Can you work these out from the model? Positions are in its coordinate system, mm. Face numbers are marked on the shaded views. A direction names the side the tool comes from. Give positions to 0.01 mm unless a question says otherwise; leave off trailing zeros. Loops run counter-clockwise (first coordinate to the right, second up) from the corner with the lowest first, then second, coordinate; pieces in that order, holes last. Notation, with made-up numbers: (83, 41.25) - (119, 41.25) arc R18 cw to (119, 50.25) - close; hole circle Ø11 at (61, 20). An arc over 180 degrees is marked (long way). Answer as a JSON object with one key per item and string values. Group by question number.
Item 1: Suppose I cut it at D-D on y = 4. Write out the boundary of the cut face in (x, z).
Item 2: Please list where these lines run through material, in increasing order: L1, parallel to Y at x = 0.5, z = 7.5; L2, parallel to Y at x = -5, z = 3.75; L3, parallel to X at y = 0, z = 8.75.
Item 3: Will these pins go through, and if not, where does the flat tip stop? pin 1 (8 mm diameter, centred on x = 14.5, y = 14, fed in from +Z); pin 2 (2 mm diameter, centred on x = -12, z = 2, fed in from +Y); pin 3 (5 mm diameter, centred on y = 20, z = 4.5, fed in from +X).
Item 4: Suppose I cut it at A-A on y = 28. Write out the boundary of the cut face in (x, z).
Item 5: Which directions (+Z, -Z, +X, -X, +Y, -Y) give clear straight access to the entire face, cutting with the end or side of a thin tool? Please do the marked faces 1, 2 and 3.
Item 6: Thinking about a two-plate mould opening in X: for the marked faces 4, 5 and 6, which applies, pulls with the +X half, pulls with the -X half, needs draft (parallel to the pull), parting line crosses it, or undercut?
Item 7: Suppose I cut it at B-B on x = 17.5. Write out the boundary of the cut face in (y, z), and give its area (3 significant figures).
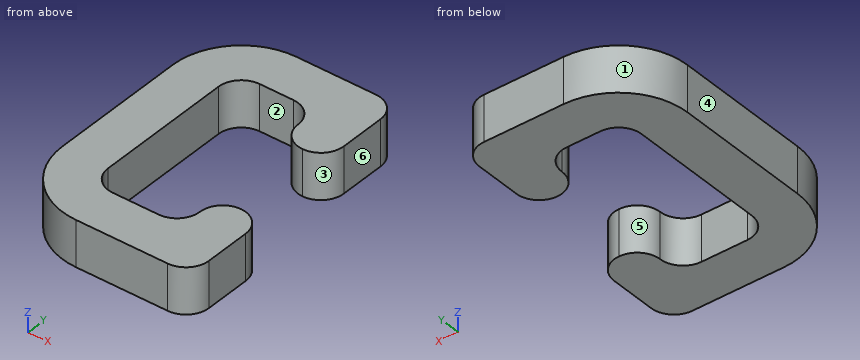
from build123d import *

# Parameters (mm, degrees)
F0_W     = 10
F0_H     = 10
F1_DEPTH = 10
F2_R     = 4.99999
F3_R     = 5
F4_R     = 5
F5_R     = 15


# Not quite as in the source:
# - a fillet or chamfer is up to 0.001 mm smaller than in the source, because OpenCascade refuses the exact size


with BuildPart() as f1:
    # F0 (on Top) → F1 (new body)
    with BuildSketch(Plane.XY):
        Polygon((10.8962109051, 41.5868479488), (10.8962109051, 31.5868479488), (10.8962109051, 21.5868479488), (20.8962109051, 21.5868479488), (20.8962109051, 41.5868479488), align=None)
        Polygon((-16.4567323537, 41.5868479488), (-16.4567323537, 31.5868479488), (-6.4567323537, 31.5868479488), (10.8962109051, 31.5868479488), (10.8962109051, 41.5868479488), align=None)
        Polygon((-6.4567323537, 31.5868479488), (-16.4567323537, 31.5868479488), (-16.4567323537, -18.4131520512), (-6.4567323537, -18.4131520512), (-6.4567323537, -8.4131520512), align=None)
        Polygon((13.5432676463, -8.4131520512), (-6.4567323537, -8.4131520512), (-6.4567323537, -18.4131520512), (23.5432676463, -18.4131520512), (23.5432676463, -8.4131520512), align=None)
        with Locations((18.5432676463, -3.4131520512)):
            Rectangle(F0_W, F0_H)
    extrude(amount=F1_DEPTH)

    # F2 (radius 5 in the source; OpenCascade refuses exactly that, so slightly less here)
    f2_edges = [f1.edges().sort_by_distance(p)[0] for p in [
        (13.543268, 1.586848, 5),
        (10.896211, 21.586848, 5),
        (10.896211, 31.586848, 5),
        (-6.456732, 31.586848, 5),
        (-6.456732, -8.413152, 5),
        (13.543268, -8.413152, 5),
    ]]
    fillet(f2_edges, radius=F2_R)

    # F3
    f3_edges = [f1.edges().sort_by_distance(p)[0] for p in [
        (23.543268, 1.586848, 5),
        (20.896211, 21.586848, 5),
    ]]
    fillet(f3_edges, radius=F3_R)

    # F4
    f4_edges = [f1.edges().sort_by_distance(p)[0] for p in [
        (23.543268, -18.413152, 5),
        (20.896211, 41.586848, 5),
    ]]
    fillet(f4_edges, radius=F4_R)

    # F5
    f5_edges = [f1.edges().sort_by_distance(p)[0] for p in [
        (-16.456732, -18.413152, 5),
        (-16.456732, 41.586848, 5),
    ]]
    fillet(f5_edges, radius=F5_R)


solid = f1.part
Worked out:
{
 "1": {"outline": "(-16.46, 0) - (-6.46, 0) - (-6.46, 10) - (-16.46, 10) - close"},
 "2": {"L1": "y = -18.41 to -8.41, 31.59 to 41.59", "L2": "y = -17.99 to -6.94, 30.11 to 41.16", "L3": "x = -16.46 to -6.46, 14.89 to 22.2"},
 "3": {"pin 1": "passes through", "pin 2": "stops at y = 38.16", "pin 3": "stops at x = 18.78"},
 "4": {"outline": "(-16.39, 0) - (-6.25, 0) - (-6.25, 10) - (-16.39, 10) - close; (10.69, 0) - (20.9, 0) - (20.9, 10) - (10.69, 10) - close"},
 "5": {"face 1": "+Z, -Z, -X, +Y", "face 2": "+Z, -Z", "face 3": "+Z, -Z, +X"},
 "6": {"face 4": "pulls with the -X half", "face 5": "undercut", "face 6": "pulls with the +X half"},
 "7": {"outline": "(-18.41, 0) - (1.48, 0) - (1.48, 10) - (-18.41, 10) - close; (21.85, 0) - (41.32, 0) - (41.32, 10) - (21.85, 10) - close", "area": "394 mm2"}
}
